Read the model definition and answer for the solid it produces. Units are mm, in the model's axes. Face numbers are marked on the shaded views. A direction names the side the tool comes from. Give positions to 0.01 mm unless a question says otherwise; leave off trailing zeros. Order: outer loops, then holes, each group sorted by start corner. A loop starts at its lowest first (then second) coordinate and runs counter-clockwise, first axis right, second up.
Item 1: A cutting plane is placed at A-A (x = 0). Write down the section's boundary in (y, z).
Item 2: A cutting plane is placed at C-C (z = -16.25). Write down the section's boundary in (x, y).
Item 3: Find the intervals of material crossed by line 1 along Y through (x, z) = (-1.75, -12.75); line 2 along Z through (x, y) = (-0.5, -3.5); line 3 along Z through (x, y) = (2, 6.25), in increasing order.
Item 4: Which of the six approach directions +Z, -Z, +X, -X, +Y, -Y give full straight-line access (tool end or side, diameter ignored) to the marked faces 1 and 2?
Item 5: A cutting plane is placed at B-B (y = 2). Write down the section's boundary in (x, z).
Item 6: A cutting plane is placed at D-D (x = 1.75). Write down the section's boundary in (y, z), plus the area to 3 significant figures.
Item 7: Given pin 1 Ø3 at (x, z) = (-2, -9) entering from -Y; pin 2 Ø3 at (x, z) = (-1.5, -6) entering from +Y, each flat-ended and moving along its own axis, determine where each tip first touches the part or whether it passes through.
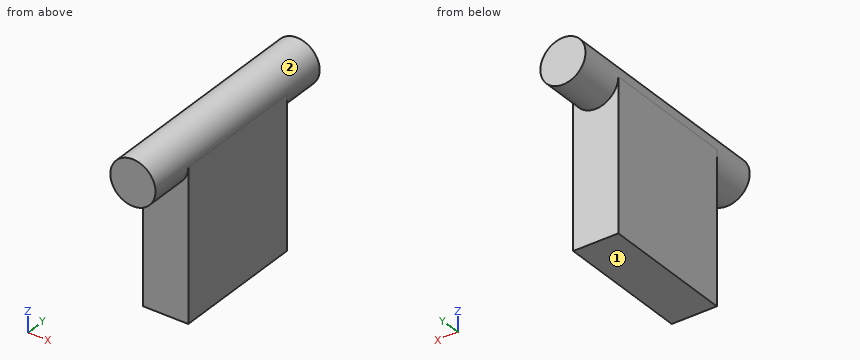
Autodesk Fusion 360 part; units mm, degrees
sketch "Sketch1" plane through (0, 0, 0) normal (0, 1, 0) x (1, 0, 0)
  circle A0 centre (0, 0) radius 3
  line L0 (2.9999, 0.0269) -> (3, 0.0269)
  line L1 (3, 0.0269) -> (3, 20)
  line L2 (3, 20) -> (-3, 20)
  line L3 (-3, 20) -> (-3, 0)
  dimension "d1" = 6
  dimension "d2" = 6
  dimension "d3" = 20
extrude "Extrude1" add sketch "Sketch1" along normal mid plane 30 contours A0 makes body 1
extrude "Extrude2" add sketch "Sketch1" along normal mid plane 18 contours A0 L1 L2 L3 bodies 1
copy_body "Body->Comp1" bodies 1 removing the originals makes body 2 in component "Component"
component "Component" placed x (1, 0, 0) y (0, 1, 0) z (0, 0, 1) at (0, 0, 0)
Response values:
1. outline: (-15, -3) - (-9, -3) - (-9, -20) - (9, -20) - (9, -3) - (15, -3) - (15, 3) - (-15, 3) - close
2. outline: (-3, -9) - (3, -9) - (3, 9) - (-3, 9) - close
3. line 1: y = -9 to 9
3. line 2: z = -20 to 2.96
3. line 3: z = -20 to 2.24
4. face 1: -Z, +X, -X, +Y, -Y
4. face 2: none
5. outline: (-3, -20) - (3, -20) - (3, -0.03) arc R3 ccw (long way) to (-3, 0) - close
6. outline: (-15, -2.44) - (-9, -2.44) - (-9, -20) - (9, -20) - (9, -2.44) - (15, -2.44) - (15, 2.44) - (-15, 2.44) - close
6. area: 462 mm2
7. pin 1: stops at y = -9
7. pin 2: stops at y = 9
